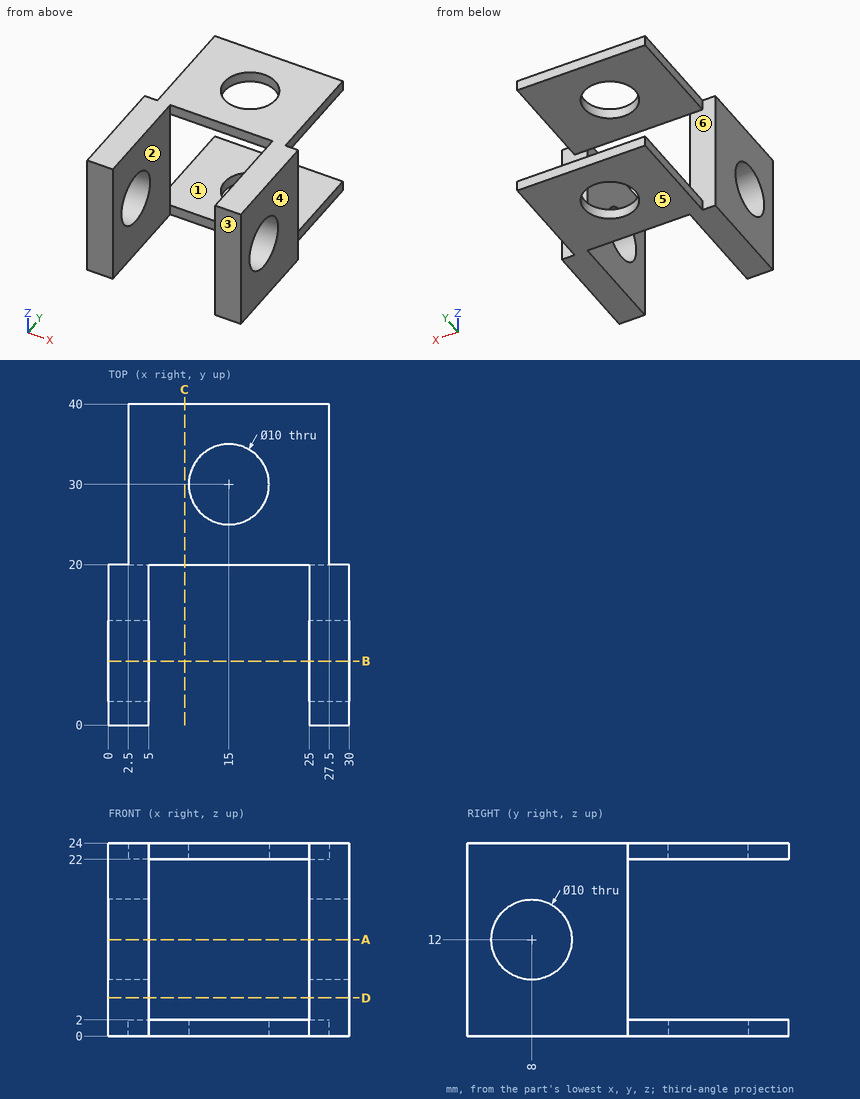
Here's the drawing with two shaded views (mm, measured from the low corner). I have some questions. A direction names the side the tool comes from. Coordinates: 2 decimals unless noted, no trailing zeros. Loops run counter-clockwise (first coordinate to the right, second up) from the corner with the lowest first, then second, coordinate; pieces in that order, holes last.
Item 1: Suppose I cut it at C-C (x = 9.5). Please give me the cut outline in (y, z), then the cut area to 3 significant figures.
Answers below:
outline: (20, 0) - (40, 0) - (40, 2) - (20, 2) - close; (20, 22) - (40, 22) - (40, 24) - (20, 24) - close
area: 80.0 mm2
Item 2: Please list where these lines run through material, in increasing order: L1, parallel to Y at x = 15, z = 23.5; L2, parallel to X at y = 18, z = 14.5; L3, parallel to Z at x = 18.25, y = 20.5.
Answers below:
L1: y = 20 to 25, 35 to 40
L2: x = 0 to 5, 25 to 30
L3: z = 0 to 2, 22 to 24
Item 3: I'm going to push flat-ended pins straight in: pin 1 (2.5 mm diameter, centred on x = 26.5, z = 10, fed in from +Y); pin 2 (1.6 mm diameter, centred on y = 26.5, z = 23, fed in from +X); pin 3 (2 mm diameter, centred on y = 33.5, z = 1, fed in from -X). Where does each tip first touch, or does it pass through?
Answers below:
pin 1: stops at y = 20
pin 2: stops at x = 27.5
pin 3: stops at x = 2.5
Item 4: Suppose I cut it at B-B (y = 8). Please give me the cut outline in (x, z), then the cut area to 3 significant figures.
Answers below:
outline: (0, 0) - (5, 0) - (5, 7) - (0, 7) - close; (0, 17) - (5, 17) - (5, 24) - (0, 24) - close; (25, 0) - (30, 0) - (30, 7) - (25, 7) - close; (25, 17) - (30, 17) - (30, 24) - (25, 24) - close
area: 140 mm2
Item 5: Suppose I cut it at A-A (z = 12). Please give me the cut outline in (x, y), then the cut area to 3 significant figures.
Answers below:
outline: (0, 0) - (5, 0) - (5, 3) - (0, 3) - close; (0, 13) - (5, 13) - (5, 20) - (0, 20) - close; (25, 0) - (30, 0) - (30, 3) - (25, 3) - close; (25, 13) - (30, 13) - (30, 20) - (25, 20) - close
area: 100 mm2
Item 6: Which directions (+Z, -Z, +X, -X, +Y, -Y) give clear straight access to the entire face, cutting with the end or side of a thin tool? Please do the marked faces 1, 2 and 3.
Answers below:
face 1: +X, -X, +Y
face 2: +Z, -Z, -Y
face 3: +Z, -Z, +X, -X, -Y
Item 7: If we mould it in two halves opening along Z, with no side actions, what happens to the marked faces 4, 5 and 6? For each: released by +Z, released by -Z, zero draft, split by the parting line, or undercut.
Answers below:
face 4: zero draft
face 5: released by -Z
face 6: undercut
Item 8: Suppose I cut it at D-D (z = 4.75). Please give me the cut outline in (x, y).
Answers below:
outline: (0, 0) - (5, 0) - (5, 20) - (0, 20) - close; (25, 0) - (30, 0) - (30, 20) - (25, 20) - close
